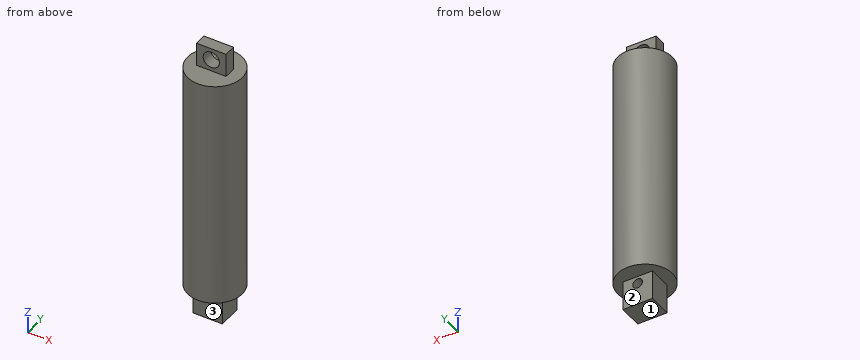
from build123d import *

# Parameters (mm, degrees)
SKETCH_1_R               = 9.25
EXTRUDE_1_DEPTH          = 78.5
SKETCH_2_W               = 10
SKETCH_2_H               = 8
EXTRUDE_2_DEPTH          = 10
SKETCH_3_W               = 10
SKETCH_3_H               = 4
EXTRUDE_3_DEPTH          = 8
CUT_EXTRUDE_1_DEPTH      = 88.996448792
CUT_EXTRUDE_1_DEPTH_BACK = 88.996448792
SKETCH_5_R               = 1.65
SKETCH_5_R_2             = 2.75


with BuildPart() as part:
    # 草图1 → 凸台-拉伸1 (new body)
    with BuildSketch(Plane.XY):
        Circle(SKETCH_1_R)
    extrude(amount=EXTRUDE_1_DEPTH)

    # 草图2 → 凸台-拉伸2 (add)
    with BuildSketch(Plane(origin=(0, 0, 0), x_dir=(-1, 0, 0), z_dir=(0, 0, -1))):
        Rectangle(SKETCH_2_W, SKETCH_2_H)
    extrude(amount=EXTRUDE_2_DEPTH)

    # 草图3 → 凸台-拉伸3 (add)
    with BuildSketch(Plane.XY.offset(78.5)):
        Rectangle(SKETCH_3_W, SKETCH_3_H)
    extrude(amount=EXTRUDE_3_DEPTH)

    # 草图5 → 切除-拉伸1 (cut, two sides: drawn at the far end of the back side and taken through both)
    with BuildSketch(Plane(origin=(0, 4, 0), x_dir=(1, 0, 0), z_dir=(0, 1, 0)).offset(-CUT_EXTRUDE_1_DEPTH_BACK)):
        with Locations(Location((0, 2.5, 0), (0, 0, 180))):
            Circle(SKETCH_5_R)
        with Locations(Location((0, -82.5, 0), (0, 0, 180))):
            Circle(SKETCH_5_R_2)
    extrude(amount=CUT_EXTRUDE_1_DEPTH + CUT_EXTRUDE_1_DEPTH_BACK, mode=Mode.SUBTRACT)


solid = part.part
Work out the finished part from the listing and answer in its coordinate system (mm). Face numbers are marked on the shaded views. A direction names the side the tool comes from. Give positions to 0.01 mm unless a question says otherwise; leave off trailing zeros. Order: outer loops, then holes, each group sorted by start corner. A loop starts at its lowest first (then second) coordinate and runs counter-clockwise, first axis right, second up. Notation, with made-up numbers: (-32.5, 29) - (-26.5, 29) arc R11 ccw to (-26.5, 39) - close; hole circle Ø10 at (67.25, -33.5). An arc over 180 degrees is marked (long way). Answer as CSV lines item,"result". Start each with the question number.
Q1. Find the intervals of material crossed by L1, parallel to Z at x = 0, y = -1; L2, parallel to X at y = 1.25, z = -2.5; L3, parallel to Z at x = 1, y = -1.25, in increasing order. Write a range as [from, to].
Q2. The part is cut by section B-B (y = 0). Write down the section's boundary in (x, z), then the cut area to 3 significant figures.
Q3. Given pin 1 Ø3 at (x, z) = (2, -7) entering from -Y; pin 2 Ø5 at (x, z) = (2, -4.5) entering from +Y; pin 3 Ø6 at (y, z) = (-4, 65.5) entering from +X, each flat-ended and moving along its own axis, determine where each tip first touches the part or whether it passes through.
Q4. The part is cut by section D-D (z = -2.5). Write down the section's boundary in (x, y), then the cut area to 3 significant figures.
Q5. The part is cut by section A-A (z = 82.5). Write down the section's boundary in (x, y), then the cut area to 3 significant figures.
Q6. For the marked faces 1, 2 and 3, determine the directions among +Z, -Z, +X, -X, +Y, -Y from which every point of the face is accessible in a straight line to the end or side of a thin tool.
Q7. The part is cut by section C-C (x = 0). Write down the section's boundary in (y, z).
Check result:
1,L1,"z = [-10, -4.15], [-0.85, 79.75], [85.25, 86.5]"
1,L2,"x = [-5, -1.65], [1.65, 5]"
1,L3,"z = [-10, -3.81], [-1.19, 79.94], [85.06, 86.5]"
2,outline,"(-9.25, 0) - (-5, 0) - (-5, -10) - (5, -10) - (5, 0) - (9.25, 0) - (9.25, 78.5) - (5, 78.5) - (5, 86.5) - (-5, 86.5) - (-5, 78.5) - (-9.25, 78.5) - close; hole circle Ø5.5 at (0, 82.5); hole circle Ø3.3 at (0, -2.5)"
2,area,"1,600 mm²"
3,pin 1,"stops at y = -4"
3,pin 2,"stops at y = 4"
3,pin 3,"stops at x = 9.2"
4,outline,"(-5, -4) - (-1.65, -4) - (-1.65, 4) - (-5, 4) - close; (1.65, -4) - (5, -4) - (5, 4) - (1.65, 4) - close"
4,area,"53.6 mm²"
5,outline,"(-5, -2) - (-2.75, -2) - (-2.75, 2) - (-5, 2) - close; (2.75, -2) - (5, -2) - (5, 2) - (2.75, 2) - close"
5,area,"18.0 mm²"
6,face 1,"-Z, +X, -X, +Y, -Y"
6,face 2,"-Z, +X, -X, +Y"
6,face 3,"-Z, +X, -X, -Y"
7,outline,"(-9.25, 0) - (-4, 0) - (-4, -0.85) - (4, -0.85) - (4, 0) - (9.25, 0) - (9.25, 78.5) - (2, 78.5) - (2, 79.75) - (-2, 79.75) - (-2, 78.5) - (-9.25, 78.5) - close; (-4, -10) - (4, -10) - (4, -4.15) - (-4, -4.15) - close; (-2, 85.25) - (2, 85.25) - (2, 86.5) - (-2, 86.5) - close"
